For this review, take the finished solid that the model builds, in its own axes (mm). Face numbers are marked on the shaded views. Give positions to 0.01 mm unless a question says otherwise; leave off trailing zeros. Write each loop counter-clockwise with the first axis right and the second up, starting at its lowest first coordinate (ties: lowest second). Pieces come first, ordered by that corner, then holes.
Q1. We need section A-A (y = 0). Write out the cut boundary in (x, z).
Q2. Mouldability with a two-part tool opening along Y and no side actions: class the marked faces 1 and 2 as released by +Y, released by -Y, zero draft, split by the parting line, or undercut.
Q3. For line 1 (Y direction, x = 6, z = 56.5); line 2 (Z direction, x = 11, y = 30); line 3 (Y direction, x = 0, z = 58.35), list the stretches that pass through material, from the lowest coordinate up.
Q4. We need section D-D (y = 20). Write out the cut boundary in (x, z), then the cut area to 3 significant figures.
Q5. Insertion check: P1, Ø3, axis at x = 5.66, y = 5.66, coming from the -Z side; P2, Ø4.5, axis at x = -5.66, y = -5.66, coming from the +Z side; P3, Ø2, axis at x = -15.5, z = 60.5, coming from the -Y side; P4, Ø3, axis at y = 2.5, z = 60, coming from the -X side. Each pin has a flat end and moves straight along its axis. Give the tip position at first contact, or say it passes through.
Q6. We need section C-C (z = 61). Write out the cut boundary in (x, y).
```python
from build123d import *

# Parameters (mm, degrees)
SKETCH001_R          = 52
SKETCH001_R_2        = 1.6
PAD001_DEPTH         = 3
SKETCH_R             = 27
SKETCH_R_2           = 24
PAD_DEPTH            = 5
SKETCH002_R          = 1.8
POCKET_DEPTH         = 5
BODY_PLACEMENT_ANGLE = 180


with BuildPart() as part:
    # Sketch001 → Pad001 (new body)
    with BuildSketch(Plane.XY):
        Circle(SKETCH001_R)
        Circle(SKETCH001_R_2, mode=Mode.SUBTRACT)
    extrude(amount=-PAD001_DEPTH)

    # Sketch → Pad (join)
    with BuildSketch(Plane.XY):
        Circle(SKETCH_R)
        Circle(SKETCH_R_2, mode=Mode.SUBTRACT)
    extrude(amount=PAD_DEPTH)

    # Sketch002 → Pocket (cut)
    with BuildSketch(Plane.XY):
        with Locations((5.656854, 5.656854)):
            Circle(SKETCH002_R)
        with Locations((-5.656854, 5.656854)):
            Circle(SKETCH002_R)
        with Locations((-5.656854, -5.656854)):
            Circle(SKETCH002_R)
        with Locations((5.656854, -5.656854)):
            Circle(SKETCH002_R)
    extrude(amount=-POCKET_DEPTH, mode=Mode.SUBTRACT)


with BuildPart() as part_1:
    # Body placement: moved
    add(part.part.moved(Location((0, 0, 59))).rotate(Axis((0, 0, 59), (0, 0, -1)), BODY_PLACEMENT_ANGLE))


solid = part_1.part
```
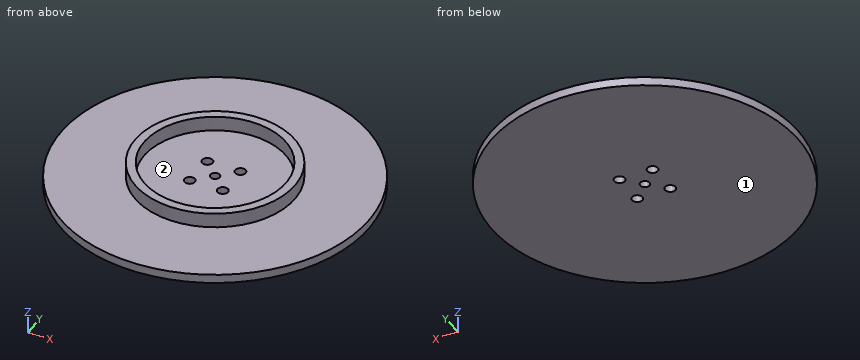
Computed:
1. outline: (-52, 56) - (-1.6, 56) - (-1.6, 59) - (-24, 59) - (-24, 64) - (-27, 64) - (-27, 59) - (-52, 59) - close; (1.6, 56) - (52, 56) - (52, 59) - (27, 59) - (27, 64) - (24, 64) - (24, 59) - (1.6, 59) - close
2. face 1: zero draft
2. face 2: undercut
3. line 1: y = -51.65 to -7.42, -3.89 to 3.89, 7.42 to 51.65
3. line 2: z = 56 to 59
3. line 3: y = -52 to -1.6, 1.6 to 52
4. outline: (-48, 56) - (48, 56) - (48, 59) - (18.14, 59) - (18.14, 64) - (13.27, 64) - (13.27, 59) - (-13.27, 59) - (-13.27, 64) - (-18.14, 64) - (-18.14, 59) - (-48, 59) - close
4. area: 337 mm2
5. P1: passes through
5. P2: stops at z = 59
5. P3: stops at y = -22.78
5. P4: stops at x = -51.98
6. outline: circle Ø54 at (0, 0); hole circle Ø48 at (0, 0)
